Verification items for the finished model (mm, model axes). A direction names the side the tool comes from. Coordinates: 2 decimals unless noted, no trailing zeros. Order: outer loops, then holes, each group sorted by start corner. A loop starts at its lowest first (then second) coordinate and runs counter-clockwise, first axis right, second up. Notation, with made-up numbers: (-10, 28) -> (10, 28) arc R14 cw to (10, 33) -> close; hole circle Ø8 at (30.25, 75). An arc over 180 degrees is marked (long way). Write each question's results on one line, items separated by ' | '. Start each with the question number.
(1) Go/stop test with flat-tipped pins: pin 1 (4 mm diameter, centred on x = 7.5, y = 24.5, fed in from +Z); pin 2 (8 mm diameter, centred on x = 4.5, z = 7, fed in from -Y); pin 3 (6 mm diameter, centred on x = 11, y = 118, fed in from -Z). Record where each tip stops, or that it passes through.
(2) Cross-section at D-D on z = 38.5. Enter the section's corners in (x, y).
(3) Set-up check for faces 5 (the flat face through (13, 130, 38)), 6 (the flat face through (13, 5, 21)), 7 (the flat face through (13, 105, 16)), 8 (the flat face through (12, 0, 16)), 9 (the flat face through (12, 53, 0)): record each of +Z, -Z, +X, -X, +Y, -Y from which the full face is reachable in a straight line by a thin tool's end or side.
(4) Cross-section at C-C on z = 13.5. Enter the section's corners in (x, y).
(5) Draft check along Y on faces 1 (the flat face through (25, 46, 4)), 2 (the cylindrical face through (12.68, 0.86, 0.9)), 3 (the flat face through (13, 100, 21)), 4 (the flat face through (12, 53, 5)). Enter one of: +Y half, -Y half, draft (parallel to the pull), parting line (faces both ways), or undercut.
(6) Thickness scan on probe 1 along Y at (x, z) = (12.5, 37.1); probe 2 along Y at (x, z) = (3.5, 24.5); probe 3 along Y at (x, z) = (7.75, 36.5). Record the ranges inside material, lowest first. Write a range as [from, to].
(7) Cross-section at B-B on x = 12.5. Enter the section's corners in (y, z), and give its area (3 significant figures).
(8) Cross-section at A-A on y = 115. Enter the section's corners in (x, z).
Autodesk Fusion 360 part; units mm, degrees
sketch "Boceto1" plane through (0, 0, 0) normal (0, 1, 0) x (1, 0, 0)
sketch "Boceto2" plane through (0, 0, 0) normal (0, 0, 1) x (1, 0, 0)
  line L0 (0, 0) -> (0, 90)
  line L1 (0, 90) -> (25, 90)
  line L2 (0, 0) -> (25, 0)
  line L3 (25, 0) -> (25, 90)
  line L4 (25, 90) -> (25, 92)
  line L5 (25, 90) -> (25, 105)
  line L6 (25, 105) -> (0, 105)
  line L7 (0, 105) -> (0, 90)
  dimension "d1" = 90
  dimension "d2" = 25
  dimension "d4" = 15
extrude "Extruir1" add sketch "Boceto2" along normal blind 5
sketch "Boceto3" plane through (0, 0, 5) normal (0, 0, 1) x (1, 0, 0)
  line L0 (0, 0) -> (25, 0)
  line L1 (25, 0) -> (25, 105)
  line L2 (25, 105) -> (0, 105)
  line L3 (0, 105) -> (0, 0)
  line L4 (0, 0) -> (25, 0)
  line L5 (25, 0) -> (25, 5)
  line L6 (25, 5) -> (0, 5)
  line L7 (0, 5) -> (0, 0)
  line L8 (0, 105) -> (25, 105)
  line L9 (25, 105) -> (25, 100)
  line L10 (25, 100) -> (0, 100)
  line L11 (0, 100) -> (0, 105)
  dimension "d7" = 5
  dimension "d8" = 5
extrude "Extruir2" add sketch "Boceto3" along normal blind 35 contours L0 L1 L3 L4 L5 L6 L7 | L1 L2 L3 L8 L9 L10 L11
sketch "Boceto4" plane through (0, 0, 0) normal (0, 1, 0) x (1, 0, 0)
  line L0 (0, -40) -> (25, -40)
  line L1 (25, -40) -> (25, -35)
  line L2 (25, -35) -> (0, -35)
  line L3 (0, -35) -> (0, -40)
  dimension "d11" = 5
extrude "Extruir3" add sketch "Boceto4" against normal blind 25
sketch "Boceto5" plane through (0, 105, 0) normal (0, 1, 0) x (-1, 0, 0)
  line L0 (-25, 0) -> (0, 0)
  line L1 (0, 0) -> (0, 40)
  line L2 (0, 40) -> (-25, 40)
  line L3 (-25, 40) -> (-25, 0)
  line L4 (-25, 40) -> (0, 40)
  line L5 (0, 40) -> (0, 35)
  line L6 (0, 35) -> (-25, 35)
  line L7 (-25, 35) -> (-25, 40)
extrude "Extruir4" add sketch "Boceto5" along normal blind 25 contours L1 L2 L3 L4 L5 L6 L7
sketch "Boceto6" plane through (0, 0, 40) normal (0, 0, 1) x (1, 0, 0)
  line L0 (0, 100) -> (25, 100)
  line L1 (25, 100) -> (25, 130)
  line L2 (25, 130) -> (0, 130)
  line L3 (0, 130) -> (0, 100)
  line L4 (12.5, 130) -> (12.5, 115)
  circle A0 centre (12.5, 115) radius 1.75
  line L5 (0, 50) -> (30, 50)
  line L6 (0, -25) -> (25, -25)
  line L7 (12.5, -25) -> (12.5, -10)
  circle A1 centre (12.5, -10) radius 1.75
  dimension "d16" = 3.5
  dimension "d17" = 3.5
extrude "Extruir5" cut sketch "Boceto6" against normal blind 5 contours A0 | A1
fillet "Empalme1" radius 5 1 edges at (12.5, 105, 35)
fillet "Empalme2" radius 5 1 edges at (12.5, 0, 35)
fillet "Empalme3" radius 3 4 edges at (12.5, 0, 0) (12.5, 105, 0) (12.5, 100, 40) (12.5, 5, 40)
fillet "Empalme4" radius 1 2 edges at (12.5, 5, 5) (12.5, 100, 5)
Results are:
1) pin 1: stops at z = 5 | pin 2: stops at y = 0 | pin 3: stops at z = 35
2) outline: (0, -25) -> (25, -25) -> (25, 4.6) -> (0, 4.6) -> close; (0, 100.4) -> (25, 100.4) -> (25, 130) -> (0, 130) -> close; hole circle Ø3.5 at (12.5, -10); hole circle Ø3.5 at (12.5, 115)
3) face 5: +Z, -Z, +X, -X, +Y | face 6: +Z, +X, -X | face 7: -Z, +X, -X, +Y | face 8: -Z, +X, -X, -Y | face 9: -Z, +X, -X, +Y, -Y
4) outline: (0, 0) -> (25, 0) -> (25, 5) -> (0, 5) -> close; (0, 100) -> (25, 100) -> (25, 105) -> (0, 105) -> close
5) face 1: draft | face 2: -Y half | face 3: undercut | face 4: undercut
6) probe 1: y = [-25, -11.75], [-8.25, 5], [100, 113.25], [116.75, 130] | probe 2: y = [0, 5], [100, 105] | probe 3: y = [-25, 5], [100, 130]
7) outline: (-25, 35) -> (-11.75, 35) -> (-11.75, 40) -> (-25, 40) -> close; (-8.25, 35) -> (-5, 35) arc R5 cw to (0, 30) -> (0, 3) arc R3 ccw to (3, 0) -> (102, 0) arc R3 ccw to (105, 3) -> (105, 30) arc R5 cw to (110, 35) -> (113.25, 35) -> (113.25, 40) -> (103, 40) arc R3 ccw to (100, 37) -> (100, 6) arc R1 cw to (99, 5) -> (6, 5) arc R1 cw to (5, 6) -> (5, 37) arc R3 ccw to (2, 40) -> (-8.25, 40) -> close; (116.75, 35) -> (130, 35) -> (130, 40) -> (116.75, 40) -> close | area: 1,090 mm2
8) outline: (0, 35) -> (10.75, 35) -> (10.75, 40) -> (0, 40) -> close; (14.25, 35) -> (25, 35) -> (25, 40) -> (14.25, 40) -> close
